Source: CAD feature listing. Evaluate the final solid. Frame: model axes, mm. Give positions to 0.01 mm unless a question says otherwise; leave off trailing zeros. Loops run counter-clockwise (first coordinate to the right, second up) from the corner with the lowest first, then second, coordinate; pieces in that order, holes last. Notation, with made-up numbers: (72.25, -1.75) -> (99.25, -1.75) arc R31 ccw to (99.25, 27.25) -> close; hole circle Ø5 at (43.25, 17.25). An arc over 180 degrees is marked (long way). Put each result on its own line as item: value.
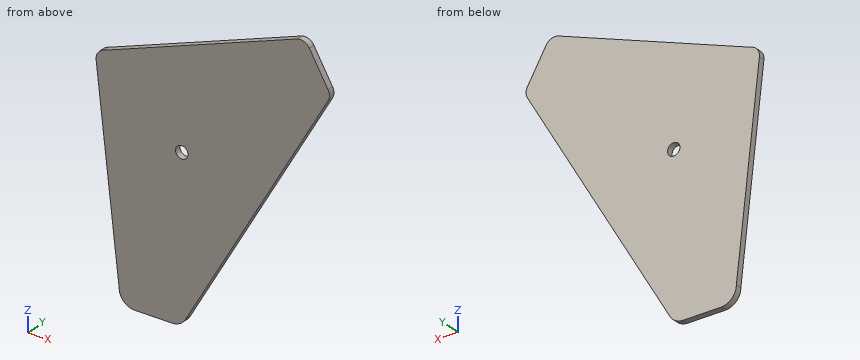
```python
from build123d import *

# Parameters (mm, degrees)
SKETCH1_R           = 6
BOSS_EXTRUDE1_DEPTH = 6


with BuildPart() as part:
    # Sketch1 → Boss-Extrude1 (new body)
    with BuildSketch(Plane.XZ):
        with BuildLine():
            Line((633.54016476, -538), (596.941268489, -538.01196066))
            ThreePointArc((596.941268489, -538.01196066), (586.334666771, -533.618562378), (581.941268489, -523.01196066))
            Line((581.941268489, -523.01196066), (559.709119696, -326.819235636))
            ThreePointArc((559.709119696, -326.819235636), (561.462040963, -319.946040825), (567.332363616, -315.964476832))
            Line((567.332363616, -315.964476832), (753.41040417, -246.551436819))
            ThreePointArc((753.41040417, -246.551436819), (760.286617927, -246.509729538), (765.564086289, -250.917947183))
            Line((765.564086289, -250.917947183), (783.574274063, -282.088977586))
            ThreePointArc((783.574274063, -282.088977586), (784.915653972, -287.088539485), (783.577542101, -292.088977052))
            Line((783.577542101, -292.088977052), (646.316882655, -530.010943959))
            ThreePointArc((646.316882655, -530.010943959), (641.004531543, -535.726307145), (633.54016476, -538))
        make_face()
        with Locations((642.330973066, -382.939920306)):
            Circle(SKETCH1_R, mode=Mode.SUBTRACT)
    extrude(amount=BOSS_EXTRUDE1_DEPTH)


solid = part.part
```
(1) Section C-C on x = 712. Return loops of the section in (y, z), then the cut area to 3 significant figures.
Calculated:
outline: (-6, -416.16) -> (0, -416.16) -> (0, -262) -> (-6, -262) -> close
area: 925 mm²
(2) Section A-A on y = -0.9. Return loops of the section in (x, z), then the cut area to 3 significant figures.
Calculated:
outline: (559.71, -326.82) -> (581.94, -523.01) arc R15 ccw to (596.94, -538.01) -> (633.54, -538) arc R15 ccw to (646.32, -530.01) -> (783.58, -292.09) arc R10 ccw to (783.57, -282.09) -> (765.56, -250.92) arc R10 ccw to (753.41, -246.55) -> (567.33, -315.96) arc R10 ccw to start; hole circle Ø12 at (642.33, -382.94)
area: 37,800 mm²
(3) First-contact query: P1, Ø6, axis at x = 650.5, z = -423, coming from the +Y side; P2, Ø1, axis at x = 711.5, y = -1, coming from the -Z side. Flat tips, straight axial feed; report the tip coordinate or a pass-through.
Calculated:
P1: stops at y = 0
P2: stops at z = -417.89
(4) Section B-B on z = -473.5. Return loops of the section in (x, y), then the cut area to 3 significant figures.
Calculated:
outline: (576.33, -6) -> (678.92, -6) -> (678.92, 0) -> (576.33, 0) -> close
area: 616 mm²
(5) Line query: probe 1 along X at (y, z) = (-5.15, -388); probe 2 along Z at (x, y) = (712.5, -0.95); probe 3 along Z at (x, y) = (734, -1.9). Output: solid intervals per line, ascending. Write a range as from..to.
Calculated:
probe 1: x = 566.64..639.11, 645.56..728.25
probe 2: z = -415.29..-261.81
probe 3: z = -378.02..-253.79
